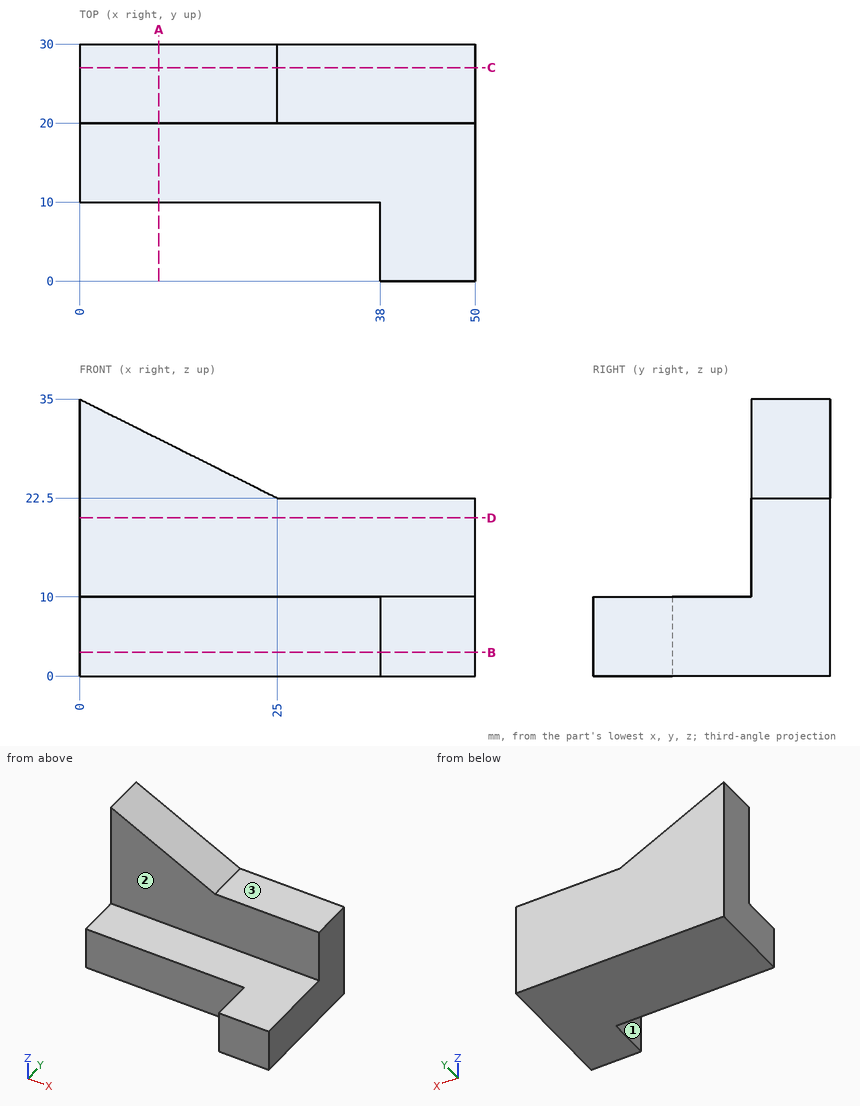
Design review of the part shown in the three views and the two pictorial views. Dimensions are in mm from the part's minimum x, y and z. A direction names the side the tool comes from. Coordinates: 2 decimals unless noted, no trailing zeros. Loops run counter-clockwise (first coordinate to the right, second up) from the corner with the lowest first, then second, coordinate; pieces in that order, holes last.
(1) Consider section B-B, the plane z = 3. Give the boundary of the cut face in (x, y), plus the area to 3 significant figures.
Determined:
outline: (0, 10) - (38, 10) - (38, 0) - (50, 0) - (50, 30) - (0, 30) - close
area: 1,120 mm2
(2) Tool access review of the marked faces 1, 2 and 3: name each direction out of +Z, -Z, +X, -X, +Y, -Y from which nothing blocks a thin tool from reaching the whole face with its end or side.
Determined:
face 1: +Z, -Z, -X, -Y
face 2: +Z, +X, -X, -Y
face 3: +Z, +X, +Y, -Y
(3) Consider section C-C, the plane y = 27. Give the boundary of the cut face in (x, z), plus the area to 3 significant figures.
Determined:
outline: (0, 0) - (50, 0) - (50, 22.5) - (25, 22.5) - (0, 35) - close
area: 1,280 mm2
(4) Wall thickness on L1, parallel to Z at x = 20, y = 27; L2, parallel to Z at x = 5.5, y = 13.25; L3, parallel to Y at x = 11.5, z = 9.5: over which ranges is each line inside the solid? List them lowest first.
Determined:
L1: z = 0 to 25
L2: z = 0 to 10
L3: y = 10 to 30
(5) Insertion check: P1, Ø5, axis at x = 36.5, y = 5, coming from the +Z side; P2, Ø12.5, axis at x = 32.5, z = 25, coming from the -Y side; P3, Ø11, axis at y = 3.5, z = 7, coming from the -X side. Each pin has a flat end and moves straight along its axis. Give the tip position at first contact, or say it passes through.
Determined:
P1: stops at z = 10
P2: stops at y = 20
P3: stops at x = 38
(6) Consider section D-D, the plane z = 20. Give the boundary of the cut face in (x, y), plus the area to 3 significant figures.
Determined:
outline: (0, 20) - (50, 20) - (50, 30) - (0, 30) - close
area: 500 mm2
(7) Consider section A-A, the plane x = 10. Give the boundary of the cut face in (y, z), plus the area to 3 significant figures.
Determined:
outline: (10, 0) - (30, 0) - (30, 30) - (20, 30) - (20, 10) - (10, 10) - close
area: 400 mm2
